Can you work these out from the model? Positions are in its coordinate system, mm. A direction names the side the tool comes from. Round coordinates to 2 decimals unless told otherwise and drop trailing zeros. Write each loop counter-clockwise with the first axis right and the second up, starting at its lowest first coordinate (ties: lowest second). Pieces come first, ordered by that corner, then holes. Notation, with made-up numbers: (60.25, 6.5) - (69.25, 6.5) arc R21 cw to (69.25, 32.5) - close; hole circle Ø5 at (63.5, -28). An arc over 180 degrees is marked (long way). One line per item, written item: value. Start each with the question number.
(1) On a 3-axis mill with a long thin cutter (end or side, diameter ignored), from which of +Z, -Z, +X, -X, +Y, -Y can I reach the whole of each face in a straight line? I mean faces 4 (the face through (29.971, -19, 0)), 5 (the face through (45.729, -35, 0)). Say none if no direction works.
(2) I want a section at C-C on z = 8.25. List the corners of the cut face in (x, y) for me.
(3) I want a section at D-D on x = 13. List the corners of the cut face in (y, z) for me, plus the area to 3 significant figures.
(4) If I drill on L1, parallel to Y at x = 32.5, z = 7.5; L2, parallel to X at y = -41.5, z = -1.5; L3, parallel to X at y = -22.5, z = 0, over which ranges is the centre line in solid material (lowest first)? Write a range as from..to.
(5) Thinking about a two-plate mould opening in Y: for faces 1 (the face through (35.729, -42, 0)), 2 (the face through (23.404, -55.873, 0.175)), 3 (the face through (9.595, -52, 0)), which applies, +Y half, -Y half, draft (parallel to the pull), parting line (faces both ways), or undercut?
(6) I want a section at B-B on x = 18.5. List the corners of the cut face in (y, z) for me.
(7) I want a section at A-A on z = -1. List the corners of the cut face in (x, y) for me.
(8) I'm going to push flat-ended pins straight in: pin 1 Ø3 at (y, z) = (-36.5, -4) entering from -X; pin 2 Ø2 at (x, z) = (31.5, 8.5) entering from -Y; pin 3 Ø8 at (x, y) = (33.5, -33.5) entering from -Z. Where does each tip first touch, or does it pass through?
from build123d import *

# Parameters (mm, degrees)
BOSS_EXTRUDE1_DEPTH = 12.5
BOSS_EXTRUDE2_DEPTH = 5.757359
FILLET2_R           = 2


with BuildPart() as part:
    # Sketch2 → Boss-Extrude1 (new, symmetric)
    with BuildSketch(Plane.XY):
        Polygon((29.971417786, -11.489425512), (29.971417786, -34.989425512), (35.728777099, -34.989425512), (35.728777099, -47.37854209), (9.594776891, -49.66497084), (9.594776891, -54.66497084), (35.728777099, -56.951399591), (45.728777099, -56.951399591), (45.728777099, -11.489425512), align=None)
    extrude(amount=BOSS_EXTRUDE1_DEPTH, both=True)

    # Sketch4 → Boss-Extrude2 (add)
    with BuildSketch(Plane.ZY.offset(-35.728777099)):
        with BuildLine():
            Line((-12.5, -34.989425512), (-12.5, -47.37854209))
            Line((-12.5, -47.37854209), (-12.499508185, -47.37854209))
            ThreePointArc((-12.499508185, -47.37854209), (-8.79954425, -38.611474116), (-6.3e-08, -34.989425512))
            Line((-6.3e-08, -34.989425512), (-12.5, -34.989425512))
        make_face()
        with BuildLine():
            Line((12.5, -34.989425512), (-6.3e-08, -34.989425512))
            ThreePointArc((-6.3e-08, -34.989425512), (8.799544205, -38.611474071), (12.499508185, -47.37854209))
            Line((12.499508185, -47.37854209), (12.5, -47.37854209))
            Line((12.5, -47.37854209), (12.5, -34.989425512))
        make_face()
    extrude(amount=BOSS_EXTRUDE2_DEPTH)

    # Sketch3 → Cut-Revolve1 (revolve, cut)
    with BuildSketch(Plane.ZY.offset(-25.728777099)):
        with BuildLine():
            Line((-12.5, -30.489425512), (12.5, -30.489425512))
            Line((12.5, -30.489425512), (12.5, -12.489425512))
            ThreePointArc((12.5, -12.489425512), (0, -24.989425512), (-12.5, -12.489425512))
            Line((-12.5, -12.489425512), (-12.5, -30.489425512))
        make_face()
    revolve(axis=Axis((25.728777099, -30.489425512, -12.5), (0, 0, 1)), mode=Mode.SUBTRACT)

    # Fillet2
    fillet2_edges = [part.edges().sort_by_distance(p)[0] for p in [
        (29.971417786, -11.489425512, 0),
        (9.594776891, -49.66497084, 0),
        (9.594776891, -54.66497084, 0),
    ]]
    fillet(fillet2_edges, radius=FILLET2_R)


solid = part.part
Established:
1. face 4: +Z, -Z, -X, +Y
1. face 5: +Z, -Z, +X, +Y, -Y
2. outline: (9.59, -52.83) arc R2 ccw to (11.42, -54.82) - (35.73, -56.95) - (45.73, -56.95) - (45.73, -11.49) - (31.97, -11.49) arc R2 ccw to (29.97, -13.49) - (29.97, -23) arc R8.61 cw to (29.97, -37.98) - (29.97, -38.1) - (35.73, -38.1) - (35.73, -47.38) - (11.42, -49.51) arc R2 ccw to (9.59, -51.5) - close
3. outline: (-54.96, -12.5) - (-49.37, -12.5) - (-49.37, 12.5) - (-54.96, 12.5) - close
3. area: 140 mm2
4. L1: -56.67..-47.66, -37.49..-34.75, -26.23..-11.49
4. L2: 35.73..45.73
4. L3: 29.97..45.73
5. face 1: undercut
5. face 2: -Y half
5. face 3: draft
6. outline: (-55.44, -12.5) - (-48.89, -12.5) - (-48.89, 12.5) - (-55.44, 12.5) - close
7. outline: (9.59, -52.83) arc R2 ccw to (11.42, -54.82) - (35.73, -56.95) - (45.73, -56.95) - (45.73, -11.49) - (31.97, -11.49) arc R2 ccw to (29.97, -13.49) - (29.97, -26.93) arc R5.54 cw to (29.97, -34.05) - (29.97, -35.03) - (35.73, -35.03) - (35.73, -47.38) - (11.42, -49.51) arc R2 ccw to (9.59, -51.5) - close
8. pin 1: x = 29.97
8. pin 2: y = -56.67
8. pin 3: z = -11.14
